Study the drawing (mm; zero at the part's minimum x, y, z) and answer. A direction names the side the tool comes from. Coordinates: 2 decimals unless noted, no trailing zeros. Loops run counter-clockwise (first coordinate to the right, second up) from the corner with the lowest first, then second, coordinate; pieces in that order, holes last. Notation, with made-up numbers: (-17, 44.5) -> (22, 44.5) arc R28 ccw to (22, 78.5) -> close; hole circle Ø8 at (-29, 40.5). An arc over 180 degrees is marked (long way). Answer as CSV lines item,"result".
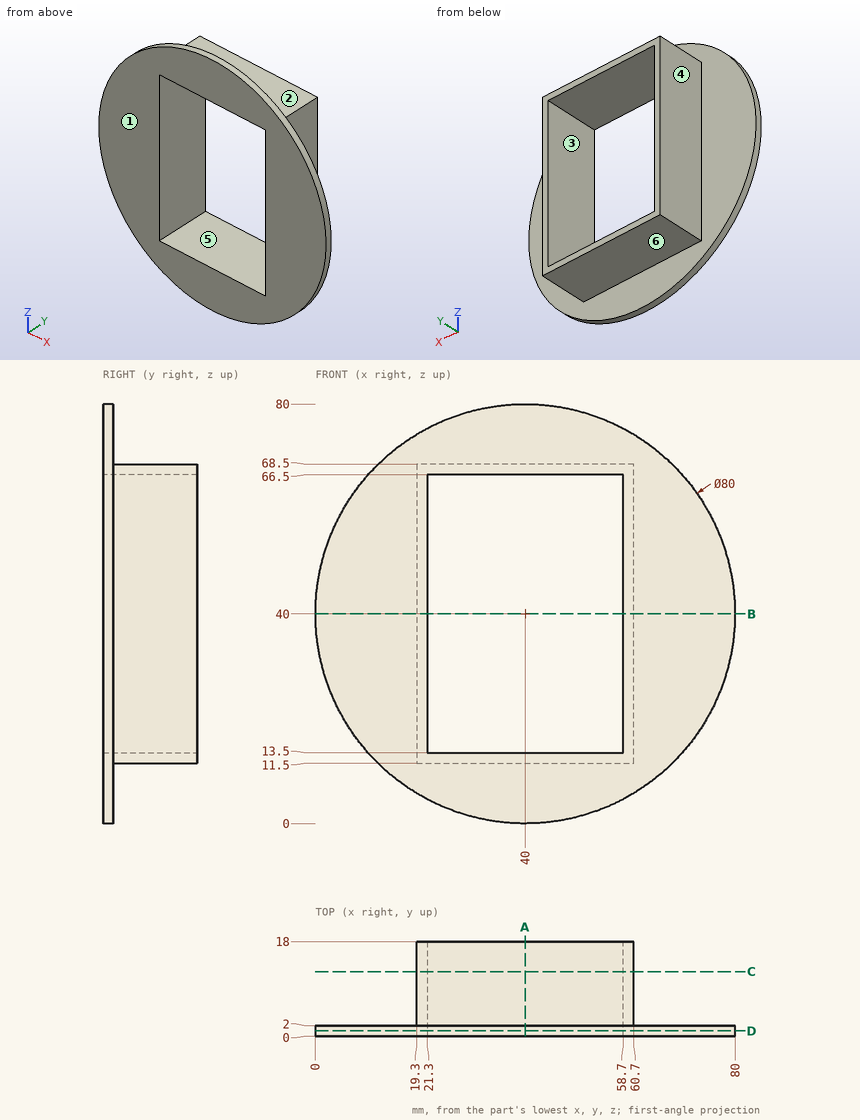
Q1. A cutting plane is placed at C-C, the plane y = 12.25. Write down the section's boundary in (x, z).
Results:
outline,"(19.3, 11.5) -> (60.7, 11.5) -> (60.7, 68.5) -> (19.3, 68.5) -> close; hole (21.3, 13.5) -> (58.7, 13.5) -> (58.7, 66.5) -> (21.3, 66.5) -> close"
Q2. A cutting plane is placed at B-B, the plane z = 40. Write down the section's boundary in (x, y), and give its area (3 significant figures).
Results:
outline,"(0, 0) -> (21.3, 0) -> (21.3, 18) -> (19.3, 18) -> (19.3, 2) -> (0, 2) -> close; (58.7, 0) -> (80, 0) -> (80, 2) -> (60.7, 2) -> (60.7, 18) -> (58.7, 18) -> close"
area,"149 mm²"
Q3. Given pin 1 Ø5.5 at (x, y) = (38, 5.5) entering from -Z; pin 2 Ø5 at (y, z) = (3, 25.5) entering from +X; pin 3 Ø8 at (y, z) = (2, 18.5) entering from -X; pin 4 Ø6 at (x, z) = (16, 42.5) entering from -Y, each flat-ended and moving along its own axis, determine where each tip first touches the part or whether it passes through.
Results:
pin 1,"stops at z = 11.5"
pin 2,"stops at x = 78.09"
pin 3,"stops at x = 4.03"
pin 4,"stops at y = 0"
Q4. A cutting plane is placed at D-D, the plane y = 1. Write down the section's boundary in (x, z), and give its area (3 significant figures).
Results:
outline,"circle Ø80 at (40, 40); hole (21.3, 13.5) -> (58.7, 13.5) -> (58.7, 66.5) -> (21.3, 66.5) -> close"
area,"3,040 mm²"
Q5. For a pull along Z with two mould halves and no side action, classify the marked faces 1, 2 and 3 as pulls with the +Z half, pulls with the -Z half, needs draft (parallel to the pull), parting line crosses it, or undercut.
Results:
face 1,"needs draft"
face 2,"pulls with the +Z half"
face 3,"undercut"
Q6. A cutting plane is placed at A-A, the plane x = 40. Write down the section's boundary in (y, z).
Results:
outline,"(0, 0) -> (2, 0) -> (2, 11.5) -> (18, 11.5) -> (18, 13.5) -> (0, 13.5) -> close; (0, 66.5) -> (18, 66.5) -> (18, 68.5) -> (2, 68.5) -> (2, 80) -> (0, 80) -> close"
Q7. Find the intervals of material crossed by probe 1 along X at (y, z) = (6.5, 59); probe 2 along Z at (x, y) = (28.5, 16.25); probe 3 along Y at (x, z) = (7, 18), in increasing order. Write a range as [from, to].
Results:
probe 1,"x = [19.3, 21.3], [58.7, 60.7]"
probe 2,"z = [11.5, 13.5], [66.5, 68.5]"
probe 3,"y = [0, 2]"
Q8. For the marked faces 4, 5 and 6, determine the directions among +Z, -Z, +X, -X, +Y, -Y from which every point of the face is accessible in a straight line to the end or side of a thin tool.
Results:
face 4,"+Z, -Z, -X, +Y"
face 5,"+Y, -Y"
face 6,"-Z, +X, -X, +Y"
